Part model, mm, in its own coordinate system. Face numbers are marked on the shaded views. A direction names the side the tool comes from. Round coordinates to 2 decimals unless told otherwise and drop trailing zeros. Loops run counter-clockwise (first coordinate to the right, second up) from the corner with the lowest first, then second, coordinate; pieces in that order, holes last. Notation, with made-up numbers: M 27,-18 L 32,-18 A30 cw 32,11 Z; hole C -8,29 d7. An arc over 180 degrees is marked long. Put each result on its own line as item: value. Start each with the question number.
1) Drop flat-ended pins along their axis: pin 1 Ø3 at (x, z) = (-18, -8) entering from +Y; pin 2 Ø6 at (x, y) = (17.5, 21) entering from -Z; pin 3 Ø2.5 at (y, z) = (21, 0.5) entering from +X. Give the stop position or say it passes through.
2) Slice it at B-B on y = 22.5. State how many separate pieces and enclosed holes the cut face has, then the cut area to 3 significant figures.
3) Slice it at A-A on x = 1. Give the cut face in (y, z), then the cut area to 3 significant figures.
4) Probe line 1 along Y through (x, z) = (39, 0); line 2 along Z through (x, y) = (-35, 6.5); line 3 along Y through (x, z) = (-35.5, 20). List the from-to ranges inside material, lowest first.
5) Which spindle directions (+Z, -Z, +X, -X, +Y, -Y) get a long thin tool onto all of the face, cutting with end or side? Do the marked faces 1, 2, 3, 4 and 5. Say none if no direction does.
```python
from build123d import *

# Parameters (mm, degrees)
SKETCH1_W                            = 85
SKETCH1_H                            = 64
BOSS_EXTRUDE1_DEPTH                  = 25.5
SKETCH2_W                            = 85
SKETCH2_H                            = 7
CUT_EXTRUDE1_DEPTH                   = 20.5
SKETCH3_W                            = 65
SKETCH3_H                            = 50
CUT_EXTRUDE2_DEPTH                   = 0.5
SKETCH4_R                            = 2.5
CUT_EXTRUDE3_DEPTH                   = 5
SKETCH5_R                            = 4
CUT_EXTRUDE4_DEPTH                   = 8
SKETCH6_R                            = 1.5
CUT_EXTRUDE5_DEPTH                   = 64
TAP_DRILL_SLOT_FOR_M3X0_5_TAP2_DEPTH = 5
TAP_START                            = 20.329155487
TAP_DRILL_SLOT_FOR_M3X0_5_TAP1_DEPTH = 4.670844513


# Read off the part's stored shape, not the designer's step: Tap Drill Slot for M3x0.5 Tap2, Tap Drill Slot for M3x0.5 Tap1
with BuildPart() as part:
    # Sketch1 → Boss-Extrude1 (new body)
    with BuildSketch(Plane(origin=(0, 0, 0), x_dir=(1, 0, 0), z_dir=(0, 1, 0))):
        Rectangle(SKETCH1_W, SKETCH1_H)
    extrude(amount=BOSS_EXTRUDE1_DEPTH)

    # Sketch2 → Cut-Extrude1 (cut)
    with BuildSketch(Plane(origin=(0, 25.5, 0), x_dir=(1, 0, 0), z_dir=(0, 1, 0))):
        with Locations((0, 28.5)):
            Rectangle(SKETCH2_W, SKETCH2_H)
        with Locations((0, -28.5)):
            Rectangle(SKETCH2_W, SKETCH2_H)
    extrude(amount=-CUT_EXTRUDE1_DEPTH, mode=Mode.SUBTRACT)

    # Sketch3 → Cut-Extrude2 (cut)
    with BuildSketch(Plane(origin=(0, 25.5, 0), x_dir=(1, 0, 0), z_dir=(0, 1, 0))):
        with Locations((-10, 0)):
            Rectangle(SKETCH3_W, SKETCH3_H)
    extrude(amount=-CUT_EXTRUDE2_DEPTH, mode=Mode.SUBTRACT)

    # Sketch4 → Cut-Extrude3 (cut)
    with BuildSketch(Plane.XY.offset(25)):
        with Locations((32.5, 15)):
            Circle(SKETCH4_R)
    extrude(amount=-CUT_EXTRUDE3_DEPTH, mode=Mode.SUBTRACT)

    # Sketch5 → Cut-Extrude4 (cut)
    with BuildSketch(Plane(origin=(42.5, 0, 0), x_dir=(0, 0, -1), z_dir=(1, 0, 0))):
        with Locations((0, 19.5)):
            Circle(SKETCH5_R)
    extrude(amount=-CUT_EXTRUDE4_DEPTH, mode=Mode.SUBTRACT)

    # Sketch6 → Cut-Extrude5 (cut)
    with BuildSketch(Plane(origin=(34.5, 0, 0), x_dir=(0, 0, -1), z_dir=(1, 0, 0))):
        with Locations((0, 19.5)):
            Circle(SKETCH6_R)
    extrude(amount=-CUT_EXTRUDE5_DEPTH, mode=Mode.SUBTRACT)

    # Tap Drill Slot for M3x0.5 Tap2 outline → Tap Drill Slot for M3x0.5 Tap2 (cut)
    with BuildSketch(Plane(origin=(0, 0, 0), x_dir=(1, 0, 0), z_dir=(0, 1, 0))):
        with BuildLine():
            Line((-38.52, -29.75), (-38.48, -29.75))
            ThreePointArc((-38.48, -29.75), (-37.23, -28.5), (-38.48, -27.25))
            Line((-38.48, -27.25), (-38.52, -27.25))
            ThreePointArc((-38.52, -27.25), (-39.77, -28.5), (-38.52, -29.75))
        make_face()
        with BuildLine():
            ThreePointArc((38.52, -29.75), (39.77, -28.5), (38.52, -27.25))
            Line((38.52, -27.25), (38.48, -27.25))
            ThreePointArc((38.48, -27.25), (37.23, -28.5), (38.48, -29.75))
            Line((38.48, -29.75), (38.52, -29.75))
        make_face()
        with BuildLine():
            Line((38.48, 27.25), (38.52, 27.25))
            ThreePointArc((38.52, 27.25), (39.77, 28.5), (38.52, 29.75))
            Line((38.52, 29.75), (38.48, 29.75))
            ThreePointArc((38.48, 29.75), (37.23, 28.5), (38.48, 27.25))
        make_face()
        with BuildLine():
            ThreePointArc((-38.48, 27.25), (-37.23, 28.5), (-38.48, 29.75))
            Line((-38.48, 29.75), (-38.52, 29.75))
            ThreePointArc((-38.52, 29.75), (-39.77, 28.5), (-38.52, 27.25))
            Line((-38.52, 27.25), (-38.48, 27.25))
        make_face()
    extrude(amount=TAP_DRILL_SLOT_FOR_M3X0_5_TAP2_DEPTH, mode=Mode.SUBTRACT)

    # Tap Drill Slot for M3x0.5 Tap1 outline → Tap Drill Slot for M3x0.5 Tap1 (cut)
    with BuildSketch(Plane(origin=(0, 0, 0), x_dir=(1, 0, 0), z_dir=(0, 1, 0)).offset(TAP_START)):
        with BuildLine():
            ThreePointArc((19.98, 1.25), (18.73, 0), (19.98, -1.25))
            Line((19.98, -1.25), (20.02, -1.25))
            ThreePointArc((20.02, -1.25), (21.27, 0), (20.02, 1.25))
            Line((20.02, 1.25), (19.98, 1.25))
        make_face()
        with BuildLine():
            ThreePointArc((13.98, 1.25), (12.73, 0), (13.98, -1.25))
            Line((13.98, -1.25), (14.02, -1.25))
            ThreePointArc((14.02, -1.25), (15.27, 0), (14.02, 1.25))
            Line((14.02, 1.25), (13.98, 1.25))
        make_face()
        with BuildLine():
            ThreePointArc((7.48, 1.25), (6.23, 0), (7.48, -1.25))
            Line((7.48, -1.25), (7.52, -1.25))
            ThreePointArc((7.52, -1.25), (8.77, 0), (7.52, 1.25))
            Line((7.52, 1.25), (7.48, 1.25))
        make_face()
        with BuildLine():
            ThreePointArc((-27.52, 1.25), (-28.77, 0), (-27.52, -1.25))
            Line((-27.52, -1.25), (-27.48, -1.25))
            ThreePointArc((-27.48, -1.25), (-26.23, 0), (-27.48, 1.25))
            Line((-27.48, 1.25), (-27.52, 1.25))
        make_face()
    extrude(amount=TAP_DRILL_SLOT_FOR_M3X0_5_TAP1_DEPTH, mode=Mode.SUBTRACT)


solid = part.part
```
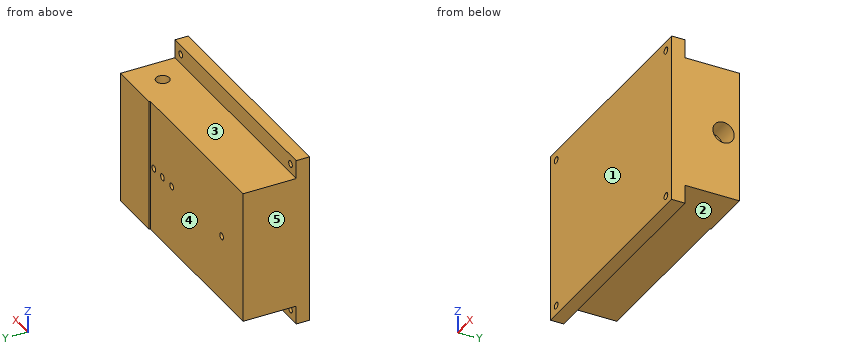
Recorded:
1. pin 1: stops at y = 25
1. pin 2: stops at z = -25
1. pin 3: stops at x = 34.5
2. separate pieces: 1
2. enclosed holes: 4
2. area: 4,190 mm2
3. outline: M 0,-32 L 5,-32 L 5,-25 L 25,-25 L 25,25 L 5,25 L 5,32 L 0,32 Z; hole C 19.5,0 d3
3. area: 1,310 mm2
4. line 1: y = 0 to 15.5, 23.5 to 25.5
4. line 2: z = -25 to 25
4. line 3: y = 0 to 25
5. face 1: +Z, -Z, +X, -X, -Y
5. face 2: -Z, +X, -X, +Y
5. face 3: +Z, +X, -X, +Y
5. face 4: +Z, -Z, -X, +Y
5. face 5: +Z, -Z, -X, +Y, -Y
